Geometry: final body of the model. Coordinates: model frame, mm. Face numbers are marked on the shaded views. Give positions to 0.01 mm unless a question says otherwise; leave off trailing zeros. One line per question, with ' | ' between items. Start each with the question number.
Autodesk Inventor part; units mm, degrees
ref_plane "YZ Plane" through (0, 0, 0) normal (1, 0, 0) x (0, 1, 0)
ref_plane "XZ Plane" through (0, 0, 0) normal (0, 1, 0) x (-1, 0, 0)
ref_plane "XY Plane" through (0, 0, 0) normal (0, 0, 1) x (1, 0, 0)
ref_plane "Work Plane1" through (-18.0552, 1.9841, 10) normal (0, 0, -1) x (-0.994, 0.1092, 0)
ref_plane "Work Plane4" through (0, 0, 10) normal (-0.994, 0.1092, 0) x (-0.1092, -0.994, 0)
ref_plane "Work Plane3" through (-40.2485, 19.0101, 10) normal (-0.994, 0.1092, 0) x (-0.1092, -0.994, 0)
sketch "Sketch1" plane through (0, 0, 10) normal (-1, 0, 0) x (0, -1, 0)
  line L0 (0, -10) -> (0, 0)
  line L1 (0, 0) -> (-65.5322, -45.8861)
  line L2 (-7.1094, 2.5876) -> (7.1094, -2.5876)
  line L3 (-65.5322, -45.8861) -> (-90.1067, -63.0934)
  dimension "d0" = 10
  dimension "d1" = 80
  dimension "d2" = 55
  dimension "d6" = 70
  dimension "d23" = 30
  dimension "d26" = 180
ref_plane "Work Plane7" through (-18.0552, 1.9841, 10) normal (0, 0, -1) x (-0.994, 0.1092, 0)
sketch "Sketch3" plane through (-18.0552, 1.9841, 10) normal (0, 0, -1) x (-0.994, 0.1092, 0)
  circle A0 centre (-18.1638, 0) radius 11.5
  circle A1 centre (-18.1638, 0) radius 2.5
  point P0 (-18.1638, 0)
  dimension "d7" = 5
sweep "Sweep1" add profiles "Sketch3" path "Sketch1" path curves L0 L1 L3 contours A1
sketch "Sketch7" plane through (0, 0, 10) normal (-1, 0, 0) x (0, -1, 0)
  line L0 (0, 0) -> (0, 0)
  line L1 (0, 0) -> (0, 0)
  line L2 (2.5, -10) -> (-2.5, -10)
  line L3 (0, 0) -> (0, 0)
  line L4 (0, 0) -> (0, 0)
  line L5 (2.5, -10) -> (2.5, 4.8025)
  line L6 (-2.5, -10) -> (-2.5, -4.8025)
  line L7 (-2.5, -4.8025) -> (0, 0)
  line L8 (0, -10) -> (0, 10)
  line L9 (4.3722, -2.276) -> (-21.1551, 11.0126)
  line L10 (-21.1551, 11.0126) -> (5.5876, 18.8192)
  line L11 (5.5876, 18.8192) -> (13.2411, 1.6857)
  line L12 (13.2411, 1.6857) -> (4.3722, -2.276)
  line L13 (-48.3403, -54.2978) -> (-48.6823, -53.3019)
  line L14 (-73.7647, -67.98) -> (-66.6763, -71.8283)
  line L15 (-66.6763, -71.8283) -> (-47.7403, -64.4229)
  line L16 (-47.7403, -64.4229) -> (-48.3403, -54.2978)
  line L17 (-55.533, -59.0685) -> (-56.5685, -56.5685)
  line L18 (-48.6823, -53.3019) -> (-76.2479, -64.72)
  line L19 (-76.2479, -64.72) -> (-73.7647, -67.98)
  point P0 (-65.0552, -65.9873)
extrude "Extrusion4" cut sketch "Sketch7" along normal mid plane 10 contours L9 L10 L11 L12
sketch "Sketch8" plane through (0, 0, 10) normal (0, -0.4617, 0.887) x (1, 0, 0)
  ellipse E0 centre (0, 0) end of major axis (0, 2.8185) minor radius 2.5 (2.5, 0) -> (-2.5, 0) ccw
  ellipse E1 centre (0, 0) end of major axis (0, -2.8185) minor radius 2.5 (-2.5, 0) -> (2.5, 0) ccw
  circle A0 centre (0, 0) radius 4.3056
  point P0 (0, -4.6175)
extrude "Extrusion5" add sketch "Sketch8" against normal blind 1 contours E1 E0 | A0
sketch "Sketch9" plane through (-6.4984, 57.0254, -46.7578) normal (0, -0.3827, -0.9239) x (0, -0.9239, 0.3827)
  ellipse E0 centre (0.4945, -6.4984) end of major axis (-6.0383, -6.4984) minor radius 2.5
  circle A0 centre (0.4945, -6.4984) radius 10.9648
  point P0 (70.578, -6.4984)
extrude "Extrusion6" [suppressed]
ref_plane "Work Plane2" through (-1.6385, -14.9102, 10) normal (0, 0, 1) x (0.994, -0.1092, 0)
properties part number "cellSTORM_lightpath"
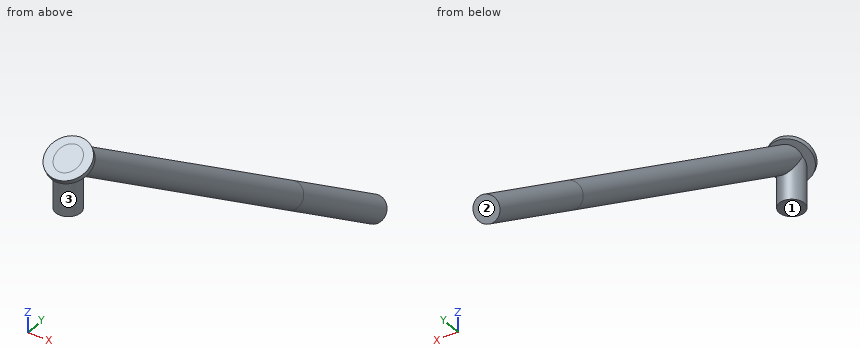
1) First-contact query: pin 1 Ø2 at (x, y) = (0, 18) entering from +Z; pin 2 Ø2.5 at (x, y) = (-0.5, 1) entering from -Z; pin 3 Ø1.5 at (x, y) = (0.5, 34) entering from -Z. Flat tips, straight axial feed; report the tip coordinate or a pass-through.
2) Pull-direction query (Y, two-part tool) for the marked faces 1, 2 and 3; classes: +Y half, -Y half, draft (parallel to the pull), parting line (faces both ways), or undercut.
3) Line query: L1, parallel to X at y = 4, z = 7; L2, parallel to Z at x = -1.5, y = 22.5; L3, parallel to Z at x = 0.75, y = 77. Output: solid intervals per line, ascending.
Answer key:
1) pin 1: z = 1.15 | pin 2: z = 0 | pin 3: z = -17.34
2) face 1: draft | face 2: +Y half | face 3: undercut
3) L1: -2.49 to 2.49 | L2: -8.2 to -3.31 | L3: -46.83 to -41.01
